Verification items for the finished model (mm, model axes). Face numbers are marked on the shaded views. A direction names the side the tool comes from. Coordinates: 2 decimals unless noted, no trailing zeros. Write each loop counter-clockwise with the first axis right and the second up, starting at its lowest first coordinate (ties: lowest second). Pieces come first, ordered by that corner, then holes. Notation, with made-up numbers: (56.25, 23.5) -> (103.25, 23.5) arc R8 ccw to (103.25, 31.5) -> close; hole circle Ø8 at (11, 80). An arc over 180 degrees is marked (long way). Answer in a Markdown table with one row per item.
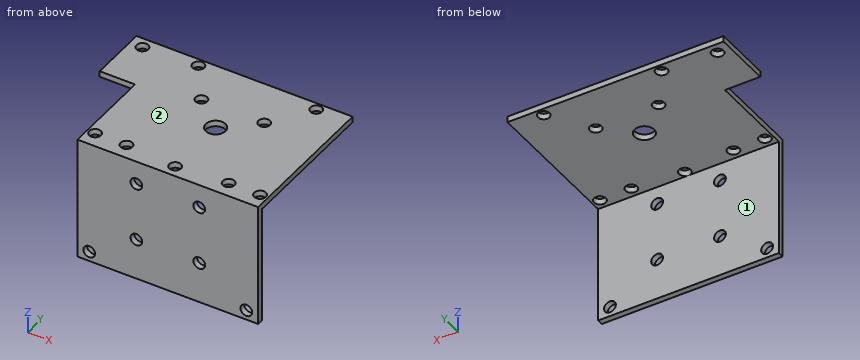
```python
from build123d import *

# Parameters (mm, degrees)
SKETCH_1_W          = 46
SKETCH_1_H          = 38.5
EXTRUDE_1_DEPTH     = 1.5
SKETCH_2_W          = 46
SKETCH_2_H          = 1.5
EXTRUDE_2_DEPTH     = 30
CUT_EXTRUDE_1_REACH = 54.896
SKETCH_3_R          = 1.5
CUT_EXTRUDE_2_REACH = 45.495
SKETCH_4_R          = 1.5
SKETCH_4_R_2        = 2.5
SKETCH_5_W          = 9
SKETCH_5_H          = 15
SKETCH_5_R          = 1.5
EXTRUDE_3_DEPTH     = 1.5


with BuildPart() as part:
    # Эскиз1 → Бобышка-Вытянуть1 (new body)
    with BuildSketch(Plane.XY):
        Rectangle(SKETCH_1_W, SKETCH_1_H)
    extrude(amount=EXTRUDE_1_DEPTH)

    # Эскиз2 → Бобышка-Вытянуть2 (add)
    with BuildSketch(Plane(origin=(0, 0, 0), x_dir=(-1, 0, 0), z_dir=(0, 0, -1))):
        with Locations((0, -18.5)):
            Rectangle(SKETCH_2_W, SKETCH_2_H)
    extrude(amount=EXTRUDE_2_DEPTH)

    # Эскиз3 → Вырез-Вытянуть1 (cut, up to next)
    with BuildSketch(Plane(origin=(0, -17.75, 0), x_dir=(1, 0, 0), z_dir=(0, 1, 0)), mode=Mode.PRIVATE) as cut_extrude_1_sk1:
        with Locations(Location((-8, 19.5, 0), (0, 0, 180))):
            Circle(SKETCH_3_R)
    cut_extrude_1_tool1 = extrude(cut_extrude_1_sk1.sketch, amount=-CUT_EXTRUDE_1_REACH, mode=Mode.PRIVATE) & part.part
    # Эскиз3 → Вырез-Вытянуть1 (cut, up to next)
    with BuildSketch(Plane(origin=(0, -17.75, 0), x_dir=(1, 0, 0), z_dir=(0, 1, 0)), mode=Mode.PRIVATE) as cut_extrude_1_sk2:
        with Locations(Location((8, 19.5, 0), (0, 0, 180))):
            Circle(SKETCH_3_R)
    cut_extrude_1_tool2 = extrude(cut_extrude_1_sk2.sketch, amount=-CUT_EXTRUDE_1_REACH, mode=Mode.PRIVATE) & part.part
    # Эскиз3 → Вырез-Вытянуть1 (cut, up to next)
    with BuildSketch(Plane(origin=(0, -17.75, 0), x_dir=(1, 0, 0), z_dir=(0, 1, 0)), mode=Mode.PRIVATE) as cut_extrude_1_sk3:
        with Locations(Location((-8, 4.5, 0), (0, 0, 180))):
            Circle(SKETCH_3_R)
    cut_extrude_1_tool3 = extrude(cut_extrude_1_sk3.sketch, amount=-CUT_EXTRUDE_1_REACH, mode=Mode.PRIVATE) & part.part
    # Эскиз3 → Вырез-Вытянуть1 (cut, up to next)
    with BuildSketch(Plane(origin=(0, -17.75, 0), x_dir=(1, 0, 0), z_dir=(0, 1, 0)), mode=Mode.PRIVATE) as cut_extrude_1_sk4:
        with Locations(Location((8, 4.5, 0), (0, 0, 180))):
            Circle(SKETCH_3_R)
    cut_extrude_1_tool4 = extrude(cut_extrude_1_sk4.sketch, amount=-CUT_EXTRUDE_1_REACH, mode=Mode.PRIVATE) & part.part
    # Эскиз3 → Вырез-Вытянуть1 (cut, up to next)
    with BuildSketch(Plane(origin=(0, -17.75, 0), x_dir=(1, 0, 0), z_dir=(0, 1, 0)), mode=Mode.PRIVATE) as cut_extrude_1_sk5:
        with Locations(Location((-20, 27.5, 0), (0, 0, 180))):
            Circle(SKETCH_3_R)
    cut_extrude_1_tool5 = extrude(cut_extrude_1_sk5.sketch, amount=-CUT_EXTRUDE_1_REACH, mode=Mode.PRIVATE) & part.part
    # Эскиз3 → Вырез-Вытянуть1 (cut, up to next)
    with BuildSketch(Plane(origin=(0, -17.75, 0), x_dir=(1, 0, 0), z_dir=(0, 1, 0)), mode=Mode.PRIVATE) as cut_extrude_1_sk6:
        with Locations(Location((20, 27.5, 0), (0, 0, 180))):
            Circle(SKETCH_3_R)
    cut_extrude_1_tool6 = extrude(cut_extrude_1_sk6.sketch, amount=-CUT_EXTRUDE_1_REACH, mode=Mode.PRIVATE) & part.part
    add(cut_extrude_1_tool1.solids().sort_by_distance((-8, -17.75, -19.5))[0], mode=Mode.SUBTRACT)
    add(cut_extrude_1_tool2.solids().sort_by_distance((8, -17.75, -19.5))[0], mode=Mode.SUBTRACT)
    add(cut_extrude_1_tool3.solids().sort_by_distance((-8, -17.75, -4.5))[0], mode=Mode.SUBTRACT)
    add(cut_extrude_1_tool4.solids().sort_by_distance((8, -17.75, -4.5))[0], mode=Mode.SUBTRACT)
    add(cut_extrude_1_tool5.solids().sort_by_distance((-20, -17.75, -27.5))[0], mode=Mode.SUBTRACT)
    add(cut_extrude_1_tool6.solids().sort_by_distance((20, -17.75, -27.5))[0], mode=Mode.SUBTRACT)

    # Эскиз4 → Вырез-Вытянуть2 (cut, up to next)
    with BuildSketch(Plane.XY.offset(1.5), mode=Mode.PRIVATE) as cut_extrude_2_sk1:
        with Locations((-15, 17.25)):
            Circle(SKETCH_4_R)
    cut_extrude_2_tool1 = extrude(cut_extrude_2_sk1.sketch, amount=-CUT_EXTRUDE_2_REACH, mode=Mode.PRIVATE) & part.part
    # Эскиз4 → Вырез-Вытянуть2 (cut, up to next)
    with BuildSketch(Plane.XY.offset(1.5), mode=Mode.PRIVATE) as cut_extrude_2_sk2:
        with Locations((15, 17.25)):
            Circle(SKETCH_4_R)
    cut_extrude_2_tool2 = extrude(cut_extrude_2_sk2.sketch, amount=-CUT_EXTRUDE_2_REACH, mode=Mode.PRIVATE) & part.part
    # Эскиз4 → Вырез-Вытянуть2 (cut, up to next)
    with BuildSketch(Plane.XY.offset(1.5), mode=Mode.PRIVATE) as cut_extrude_2_sk3:
        with Locations((-8, 7.25)):
            Circle(SKETCH_4_R)
    cut_extrude_2_tool3 = extrude(cut_extrude_2_sk3.sketch, amount=-CUT_EXTRUDE_2_REACH, mode=Mode.PRIVATE) & part.part
    # Эскиз4 → Вырез-Вытянуть2 (cut, up to next)
    with BuildSketch(Plane.XY.offset(1.5), mode=Mode.PRIVATE) as cut_extrude_2_sk4:
        with Locations(Location((8, 7.25, 0), (0, 0, 180))):
            Circle(SKETCH_4_R)
    cut_extrude_2_tool4 = extrude(cut_extrude_2_sk4.sketch, amount=-CUT_EXTRUDE_2_REACH, mode=Mode.PRIVATE) & part.part
    # Эскиз4 → Вырез-Вытянуть2 (cut, up to next)
    with BuildSketch(Plane.XY.offset(1.5), mode=Mode.PRIVATE) as cut_extrude_2_sk5:
        with Locations((0, 0.25)):
            Circle(SKETCH_4_R_2)
    cut_extrude_2_tool5 = extrude(cut_extrude_2_sk5.sketch, amount=-CUT_EXTRUDE_2_REACH, mode=Mode.PRIVATE) & part.part
    # Эскиз4 → Вырез-Вытянуть2 (cut, up to next)
    with BuildSketch(Plane.XY.offset(1.5), mode=Mode.PRIVATE) as cut_extrude_2_sk6:
        with Locations((0, -16.25)):
            Circle(SKETCH_4_R)
    cut_extrude_2_tool6 = extrude(cut_extrude_2_sk6.sketch, amount=-CUT_EXTRUDE_2_REACH, mode=Mode.PRIVATE) & part.part
    # Эскиз4 → Вырез-Вытянуть2 (cut, up to next)
    with BuildSketch(Plane.XY.offset(1.5), mode=Mode.PRIVATE) as cut_extrude_2_sk7:
        with Locations((-21, -15.25)):
            Circle(SKETCH_4_R)
    cut_extrude_2_tool7 = extrude(cut_extrude_2_sk7.sketch, amount=-CUT_EXTRUDE_2_REACH, mode=Mode.PRIVATE) & part.part
    # Эскиз4 → Вырез-Вытянуть2 (cut, up to next)
    with BuildSketch(Plane.XY.offset(1.5), mode=Mode.PRIVATE) as cut_extrude_2_sk8:
        with Locations(Location((21, -15.25, 0), (0, 0, 180))):
            Circle(SKETCH_4_R)
    cut_extrude_2_tool8 = extrude(cut_extrude_2_sk8.sketch, amount=-CUT_EXTRUDE_2_REACH, mode=Mode.PRIVATE) & part.part
    # Эскиз4 → Вырез-Вытянуть2 (cut, up to next)
    with BuildSketch(Plane.XY.offset(1.5), mode=Mode.PRIVATE) as cut_extrude_2_sk9:
        with Locations((-13, -15.25)):
            Circle(SKETCH_4_R)
    cut_extrude_2_tool9 = extrude(cut_extrude_2_sk9.sketch, amount=-CUT_EXTRUDE_2_REACH, mode=Mode.PRIVATE) & part.part
    # Эскиз4 → Вырез-Вытянуть2 (cut, up to next)
    with BuildSketch(Plane.XY.offset(1.5), mode=Mode.PRIVATE) as cut_extrude_2_sk10:
        with Locations(Location((13, -15.25, 0), (0, 0, 180))):
            Circle(SKETCH_4_R)
    cut_extrude_2_tool10 = extrude(cut_extrude_2_sk10.sketch, amount=-CUT_EXTRUDE_2_REACH, mode=Mode.PRIVATE) & part.part
    add(cut_extrude_2_tool1.solids().sort_by_distance((-15, 17.25, 1.5))[0], mode=Mode.SUBTRACT)
    add(cut_extrude_2_tool2.solids().sort_by_distance((15, 17.25, 1.5))[0], mode=Mode.SUBTRACT)
    add(cut_extrude_2_tool3.solids().sort_by_distance((-8, 7.25, 1.5))[0], mode=Mode.SUBTRACT)
    add(cut_extrude_2_tool4.solids().sort_by_distance((8, 7.25, 1.5))[0], mode=Mode.SUBTRACT)
    add(cut_extrude_2_tool5.solids().sort_by_distance((0, 0.25, 1.5))[0], mode=Mode.SUBTRACT)
    add(cut_extrude_2_tool6.solids().sort_by_distance((0, -16.25, 1.5))[0], mode=Mode.SUBTRACT)
    add(cut_extrude_2_tool7.solids().sort_by_distance((-21, -15.25, 1.5))[0], mode=Mode.SUBTRACT)
    add(cut_extrude_2_tool8.solids().sort_by_distance((21, -15.25, 1.5))[0], mode=Mode.SUBTRACT)
    add(cut_extrude_2_tool9.solids().sort_by_distance((-13, -15.25, 1.5))[0], mode=Mode.SUBTRACT)
    add(cut_extrude_2_tool10.solids().sort_by_distance((13, -15.25, 1.5))[0], mode=Mode.SUBTRACT)

    # Эскиз5 → Бобышка-Вытянуть3 (add)
    with BuildSketch(Plane(origin=(0, 0, 0), x_dir=(-1, 0, 0), z_dir=(0, 0, -1))):
        with Locations((27.5, 11.75)):
            Rectangle(SKETCH_5_W, SKETCH_5_H)
        with Locations((28.78, 16.5)):
            Circle(SKETCH_5_R, mode=Mode.SUBTRACT)
    extrude(amount=-EXTRUDE_3_DEPTH)


solid = part.part
```
1. Tool access check on the marked faces 1 and 2. Record the directions out of +Z, -Z, +X, -X, +Y, -Y that give a thin tool (end or side, any length) a straight path to the whole face; none if there is none.
Geometry says:
| item | result |
|---|---|
| face 1 | -Z, +X, -X, +Y |
| face 2 | +Z, +X, -X, +Y, -Y |
2. Section check A-A, the plane z = -19.5. Record the boundary of the cut face in (x, y), plus the area to 3 significant figures.
Geometry says:
| item | result |
|---|---|
| outline | (-23, -19.25) -> (-9.5, -19.25) -> (-9.5, -17.75) -> (-23, -17.75) -> close; (-6.5, -19.25) -> (6.5, -19.25) -> (6.5, -17.75) -> (-6.5, -17.75) -> close; (9.5, -19.25) -> (23, -19.25) -> (23, -17.75) -> (9.5, -17.75) -> close |
| area | 60.0 mm^2 |
3. Thickness scan on line 1 (Z direction, x = -8, y = -18.65); line 2 (Z direction, x = -20, y = -18.9); line 3 (Y direction, x = -13, z = 1). Record the ranges inside material, lowest first. Write a range as from..to.
Geometry says:
| item | result |
|---|---|
| line 1 | -30..-21, -18..-6, -3..1.5 |
| line 2 | -30..-29, -26..1.5 |
| line 3 | -19.25..-16.75, -13.75..19.25 |
4. Section check D-D, the plane y = 0.25. Record the boundary of the cut face in (x, z), plus the area to 3 significant figures.
Geometry says:
| item | result |
|---|---|
| outline | (-23, 0) -> (-2.5, 0) -> (-2.5, 1.5) -> (-23, 1.5) -> close; (2.5, 0) -> (23, 0) -> (23, 1.5) -> (2.5, 1.5) -> close |
| area | 61.5 mm^2 |
5. Section check C-C, the plane x = 8. Record the boundary of the cut face in (y, z).
Geometry says:
| item | result |
|---|---|
| outline | (-19.25, -30) -> (-17.75, -30) -> (-17.75, -21) -> (-19.25, -21) -> close; (-19.25, -18) -> (-17.75, -18) -> (-17.75, -6) -> (-19.25, -6) -> close; (-19.25, -3) -> (-17.75, -3) -> (-17.75, 0) -> (5.75, 0) -> (5.75, 1.5) -> (-19.25, 1.5) -> close; (8.75, 0) -> (19.25, 0) -> (19.25, 1.5) -> (8.75, 1.5) -> close |
6. Depth check by flat-ended pin: P1, Ø2.5, axis at x = 20, z = -27.5, coming from the -Y side; P2, Ø2, axis at x = 5, z = -3, coming from the +Y side; P3, Ø5, axis at x = -28.78, y = 16.5, coming from the -Z side; P4, Ø1.2, axis at x = -29.5, z = 1, coming from the -Y side. Enter the tip coordinate at first touch or a pass-through.
Geometry says:
| item | result |
|---|---|
| P1 | through |
| P2 | y = -17.75 |
| P3 | z = 0 |
| P4 | y = 4.25 |
7. Section check B-B, the plane y = 7.25. Record the boundary of the cut face in (x, z).
Geometry says:
| item | result |
|---|---|
| outline | (-32, 0) -> (-9.5, 0) -> (-9.5, 1.5) -> (-32, 1.5) -> close; (-6.5, 0) -> (6.5, 0) -> (6.5, 1.5) -> (-6.5, 1.5) -> close; (9.5, 0) -> (23, 0) -> (23, 1.5) -> (9.5, 1.5) -> close |
